from build123d import *

# Parameters (mm, degrees)
F0_W          = 8.4836
F0_H          = 3.175
F1_DEPTH      = 12.7
F3_DEPTH      = 8.89
F3_DEPTH_BACK = 3.81
F4_R          = 5.08
F5_DEPTH      = 6.35
F6_R          = 1.27
F7_DEPTH      = 25.4
F8_R          = 1.27
F9_DEPTH      = 124.4092
F10_W         = 10.82675
F10_H         = 7.62
F11_DEPTH     = 45.72
F12_W         = 44.831
F12_H         = 7.62
F13_DEPTH     = 76.2
F14_R         = 1.7145
F15_DEPTH     = 51.6382
F16_W         = 12.7
F16_H         = 14.986
F17_DEPTH     = 3.175
F18_W         = 12.7
F18_H         = 14.986
F19_DEPTH     = 3.175
F20_W         = 12.7
F20_H         = 1.778
F20_R         = 1.27
F21_DEPTH     = 51.054
F23_DEPTH     = 50.8
F24_W         = 12.7
F24_H         = 3.175
F25_DEPTH     = 22.86


with BuildPart() as f1:
    # F0 (on Front) → F1 (new body)
    with BuildSketch(Plane.XZ):
        with Locations((4.2418, 1.5875)):
            Rectangle(F0_W, F0_H)
    extrude(amount=F1_DEPTH)

    # F2 (on face) → F3 (join, two sides)
    with BuildSketch(Plane(origin=(0, 0, 0), x_dir=(-1, 0, 0), z_dir=(0, 1, 0))) as f3_sk:
        Polygon((-8.4836, 3.175), (-8.4836, 0), (-13.7668, 0), (-23.4823, 0), (-23.4823, 13.208), (-26.6573, 13.208), (-26.6573, -7.62), (-12.1793, -7.62), (-4.2418, -7.62), (3.6957, -7.62), (18.1737, -7.62), (18.1737, 13.208), (14.9987, 13.208), (14.9987, 0), (5.2832, 0), (0, 0), (0, 3.175), align=None)
    extrude(amount=F3_DEPTH)
    extrude(f3_sk.sketch, amount=-F3_DEPTH_BACK)

    # F4 (on face) → F5 (join)
    with BuildSketch(Plane.XZ.offset(12.7)):
        with BuildLine():
            Line((8.4836, 0), (8.4836, 10.59766))
            ThreePointArc((8.4836, 10.59766), (4.2418, 21.673084), (0, 10.59766))
            Line((0, 10.59766), (0, 0))
            Line((0, 0), (8.4836, 0))
        make_face()
        with Locations((4.2418, 15.323084)):
            Circle(F4_R, mode=Mode.SUBTRACT)
    extrude(amount=F5_DEPTH)

    # F6 (on face) → F7 (cut)
    with BuildSketch(Plane.XY.offset(3.175)):
        with Locations((4.2418, -6.95039)):
            Circle(F6_R)
    extrude(amount=-F7_DEPTH, mode=Mode.SUBTRACT)

    # F8 (on face) → F9 (cut)
    with BuildSketch(Plane.YZ.offset(26.6573)):
        with Locations((2.54, 5.715)):
            Circle(F8_R)
    extrude(amount=-F9_DEPTH, mode=Mode.SUBTRACT)

    # F10 (on face) → F11 (join)
    with BuildSketch(Plane(origin=(0, 8.89, 0), x_dir=(-1, 0, 0), z_dir=(0, 1, 0))):
        with Locations((-21.243925, -3.81)):
            Rectangle(F10_W, F10_H)
        with Locations((12.760325, -3.81)):
            Rectangle(F10_W, F10_H)
    extrude(amount=F11_DEPTH)

    # F12 (on face) → F13 (join)
    with BuildSketch(Plane(origin=(0, 54.61, 0), x_dir=(-1, 0, 0), z_dir=(0, 1, 0))):
        with Locations((-4.2418, -3.81)):
            Rectangle(F12_W, F12_H)
    extrude(amount=F13_DEPTH)

    # F14 (on face) → F15 (cut)
    with BuildSketch(Plane.YZ.offset(26.6573)):
        with Locations((31.75, -3.81)):
            Circle(F14_R)
    extrude(amount=-F15_DEPTH, mode=Mode.SUBTRACT)

    # F16 (on face) → F17 (join)
    with BuildSketch(Plane.YZ.offset(26.6573)):
        with Locations((76.2, 7.493)):
            Rectangle(F16_W, F16_H)
    extrude(amount=-F17_DEPTH)

    # F18 (on face) → F19 (join)
    with BuildSketch(Plane(origin=(-18.1737, 0, 0), x_dir=(0, -1, 0), z_dir=(-1, 0, 0))):
        with Locations((-76.2, 7.493)):
            Rectangle(F18_W, F18_H)
    extrude(amount=-F19_DEPTH)

    # F20 (on face) → F21 (cut)
    with BuildSketch(Plane.YZ.offset(26.6573)):
        with Locations((76.2, 14.097)):
            Rectangle(F20_W, F20_H)
        with Locations((76.2, 5.715)):
            Circle(F20_R)
    extrude(amount=-F21_DEPTH, mode=Mode.SUBTRACT)

    # F22 (on face) → F23 (cut)
    with BuildSketch(Plane(origin=(0, 130.81, 0), x_dir=(-1, 0, 0), z_dir=(0, 1, 0))):
        Polygon((-10.5918, -7.62), (-4.2418, -7.62), (2.1082, -7.62), (2.1082, -4.445), (-10.5918, -4.445), align=None)
    extrude(amount=-F23_DEPTH, mode=Mode.SUBTRACT)

    # F24 (on face) → F25 (join)
    with BuildSketch(Plane(origin=(0, 130.81, 0), x_dir=(-1, 0, 0), z_dir=(0, 1, 0))):
        with Locations((-4.2418, -6.0325)):
            Rectangle(F24_W, F24_H)
    extrude(amount=-F25_DEPTH)


solid = f1.part
Work out the finished part from the listing and answer in its coordinate system (mm). A direction names the side the tool comes from. Give positions to 0.01 mm unless a question says otherwise; leave off trailing zeros. Order: outer loops, then holes, each group sorted by start corner. A loop starts at its lowest first (then second) coordinate and runs counter-clockwise, first axis right, second up. Notation, with made-up numbers: (-16.75, 64.5) - (-3.75, 64.5) arc R22 ccw to (-3.75, 85.5) - close; hole circle Ø10 at (61.25, 46). An arc over 180 degrees is marked (long way). Answer as CSV lines item,"result". Start each with the question number.
Q1. The part is cut by section A-A (x = -5.5). Write down the section's boundary in (y, z).
Q2. The mould has two halves that part along Y. Classify faces 1 (the face through (4, 54.61, -4)), 2 (the face through (5, 130.81, -4)), 3 (the face through (25, 8.89, 7)), 4 (the face through (4.46, -15.83, 21.67)): +Y half, -Y half, draft (parallel to the pull), parting line (faces both ways), or undercut.
Q3. For faces 5 (the face through (8.484, -8, 3)), 6 (the face through (4, 107.95, -6)), 7 (the face through (-14.999, 1, 7)), 8 (the face through (25, 76, 13.208)), determine the directions among +Z, -Z, +X, -X, +Y, -Y from which every point of the face is accessible in a straight line to the end or side of a thin tool.
Q4. Given pin 1 Ø3.5 at (x, y) = (-17, 4) entering from +Z; pin 2 Ø2.5 at (x, z) = (25, 8) entering from +Y; pin 3 Ø14 at (x, z) = (5.5, 10.5) entering from +Y; pin 4 Ø1.5 at (y, z) = (76.2, 5.715) entering from +X, each flat-ended and moving along its own axis, determine where each tip first touches the part or whether it passes through.
Q5. Find the intervals of material crossed by L1, parallel to X at y = -1, z = 5.75; L2, parallel to Y at x = 14, z = -2.75; L3, parallel to Z at x = -1, y = 112, in increasing order. Write a range as [from, to].
Q6. The part is cut by section B-B (z = 1.75). Write down the section's boundary in (x, y).
Q7. The part is cut by section D-D (y = 92). Write down the section's boundary in (x, z) (3 decimals).
Q8. The part is cut by section C-C (y = 42). Write down the section's boundary in (x, z), then the cut area to 3 significant figures.
Check result:
1,outline,"(-3.81, -7.62) - (8.89, -7.62) - (8.89, 0) - (-3.81, 0) - close; (54.61, -7.62) - (130.81, -7.62) - (130.81, 0) - (54.61, 0) - close"
2,face 1,"undercut"
2,face 2,"+Y half"
2,face 3,"undercut"
2,face 4,"draft"
3,face 5,"+Y, -Y"
3,face 6,"-Z"
3,face 7,"+Z, +Y, -Y"
3,face 8,"+Z, +X, -X, +Y, -Y"
4,pin 1,"stops at z = 13.21"
4,pin 2,"stops at y = 82.55"
4,pin 3,"stops at y = -12.7"
4,pin 4,"passes through"
5,L1,"x = [-18.17, -15], [23.48, 26.66]"
5,L2,"y = [-3.81, 8.89], [54.61, 130.81]"
5,L3,"z = [-7.62, 0]"
6,outline,"(-18.17, -3.81) - (-15, -3.81) - (-15, 8.89) - (-18.17, 8.89) - close; (-18.17, 69.85) - (-15, 69.85) - (-15, 82.55) - (-18.17, 82.55) - close; (0, -19.05) - (8.48, -19.05) - (8.48, 8.89) - (0, 8.89) - close; (23.48, -3.81) - (26.66, -3.81) - (26.66, 8.89) - (23.48, 8.89) - close; (23.48, 69.85) - (26.66, 69.85) - (26.66, 82.55) - (23.48, 82.55) - close; hole circle Ø2.54 at (4.24, -6.95)"
7,outline,"(-18.174, -7.62) - (-2.108, -7.62) - (-2.108, -4.445) - (10.592, -4.445) - (10.592, -7.62) - (26.657, -7.62) - (26.657, 0) - (-18.174, 0) - close"
8,outline,"(-18.17, -7.62) - (-7.35, -7.62) - (-7.35, 0) - (-18.17, 0) - close; (15.83, -7.62) - (26.66, -7.62) - (26.66, 0) - (15.83, 0) - close"
8,area,"165 mm²"
